```python
from build123d import *

# Parameters (mm, degrees)
ESQUISSE1_R             = 28
BOSS_EXTRU_1_DEPTH      = 7
ESQUISSE2_R             = 3.8
BOSS_EXTRU_2_DEPTH      = 10
ESQUISSE3_R             = 3.05
ENL_V_MAT_EXTRU_1_DEPTH = 18
ESQUISSE4_R             = 2
ESQUISSE5_R             = 5.75
ESQUISSE5_R_2           = 3.8
BOSS_EXTRU_3_DEPTH      = 6
ENL_V_MAT_EXTRU_2_REACH = 30
ESQUISSE6_R             = 1.5


with BuildPart() as part:
    # Esquisse1 → Boss.-Extru.1 (new body)
    with BuildSketch(Plane.XY):
        Circle(ESQUISSE1_R)
    extrude(amount=BOSS_EXTRU_1_DEPTH)

    # Esquisse2 → Boss.-Extru.2 (add)
    with BuildSketch(Plane.XY.offset(7)):
        Circle(ESQUISSE2_R)
    extrude(amount=BOSS_EXTRU_2_DEPTH)

    # Esquisse3 → Enlèv. mat.-Extru.1 (cut, through all)
    with BuildSketch(Plane.XY.offset(17)):
        Circle(ESQUISSE3_R)
    extrude(amount=-ENL_V_MAT_EXTRU_1_DEPTH, mode=Mode.SUBTRACT)

    # Esquisse4 → Enlèvement de matière-Révolution1 (revolve, cut)
    with BuildSketch(Plane(origin=(0, 0, 0), x_dir=(0, 0, -1), z_dir=(1, 0, 0))):
        with Locations((-3.5, 28)):
            Circle(ESQUISSE4_R)
    revolve(axis=Axis((0, 0, 0), (0, 0, 1)), mode=Mode.SUBTRACT)

    # Esquisse5 → Boss.-Extru.3 (add)
    with BuildSketch(Plane.XY.offset(7)):
        Circle(ESQUISSE5_R)
        Circle(ESQUISSE5_R_2, mode=Mode.SUBTRACT)
    extrude(amount=BOSS_EXTRU_3_DEPTH)

    # Esquisse6 → Enlèv. mat.-Extru.2 (cut, up to next)
    with BuildSketch(Plane(origin=(0, 0, 0), x_dir=(1, 0, 0), z_dir=(0, 1, 0)), mode=Mode.PRIVATE) as enl_v_mat_extru_2_sk1:
        with Locations((0, -10)):
            Circle(ESQUISSE6_R)
    enl_v_mat_extru_2_tool1 = extrude(enl_v_mat_extru_2_sk1.sketch, amount=ENL_V_MAT_EXTRU_2_REACH, mode=Mode.PRIVATE) & part.part
    add(enl_v_mat_extru_2_tool1.solids().sort_by_distance((0, 0, 10))[0], mode=Mode.SUBTRACT)


solid = part.part
```
Read the model definition and answer for the solid it produces. Units are mm, in the model's axes. A direction names the side the tool comes from. Give positions to 0.01 mm unless a question says otherwise; leave off trailing zeros. Write each loop counter-clockwise with the first axis right and the second up, starting at its lowest first coordinate (ties: lowest second). Pieces come first, ordered by that corner, then holes. Notation, with made-up numbers: (-36, 8) -> (-28, 8) arc R22 ccw to (-28, 44) -> close; hole circle Ø5 at (84, 13). An arc over 180 degrees is marked (long way). Answer as a JSON object with one key per item and string values.
1) Flat-ended cylindrical pins translate along their axes: pin 1 Ø3.5 at (x, z) = (0, 10) entering from +Y; pin 2 Ø2 at (x, z) = (14.5, 5) entering from +Y; pin 3 Ø10 at (x, y) = (-9, -2) entering from +Z. Find the tip coordinate at first contact, or state that the pin passes through.
Findings below:
{"pin 1": "stops at y = 5.75", "pin 2": "stops at y = 24.46", "pin 3": "stops at z = 13"}
2) For a pull along X with two mould halves and no side action, classify faces 3 (the flat face through (6, 0, 0)), 4 (the cylindrical face through (26.707, 8.41, 0.74)), 5 (the cylindrical face through (1.386, 4.184, 10.575)) as pulls with the +X half, pulls with the -X half, needs draft (parallel to the pull), parting line crosses it, or undercut.
Findings below:
{"face 3": "needs draft", "face 4": "parting line crosses it", "face 5": "undercut"}
3) Straight lines are drawn through the part: probe 1 along Z at (x, y) = (0, 4); probe 2 along Z at (x, y) = (13.5, -9); probe 3 along Y at (x, z) = (0, 6.5). For each, find the intervals that lie inside material, in ascending order. Write a range as from..to.
Findings below:
{"probe 1": "z = 0..8.5, 11.5..13", "probe 2": "z = 0..7", "probe 3": "y = -28..-3.05, 3.05..28"}
4) Section B-B on x = 0 is taken. Write down the section's boundary in (y, z), then the cut area to 3 significant figures.
Findings below:
{"outline": "(-28, 0) -> (-3.05, 0) -> (-3.05, 17) -> (-3.8, 17) -> (-3.8, 13) -> (-5.75, 13) -> (-5.75, 7) -> (-28, 7) -> (-28, 5.5) arc R2 cw to (-28, 1.5) -> close; (3.05, 0) -> (28, 0) -> (28, 1.5) arc R2 cw to (28, 5.5) -> (28, 7) -> (5.75, 7) -> (5.75, 8.5) -> (3.05, 8.5) -> close; (3.05, 11.5) -> (5.75, 11.5) -> (5.75, 13) -> (3.8, 13) -> (3.8, 17) -> (3.05, 17) -> close", "area": "367 mm^2"}
5) A tool of negligible diameter and unlimited length cuts with its end or side. For faces 1 (the flat face through (1, -4, 13)), 2 (the cylindrical face through (25.865, -10.724, 6.24)), from which of +Z, -Z, +X, -X, +Y, -Y can it reach the whole face along a straight path? Write none if from no direction.
Findings below:
{"face 1": "+Z", "face 2": "+Z, -Z"}
6) Section A-A on y = 0 is taken. Write down the section's boundary in (x, z).
Findings below:
{"outline": "(-28, 0) -> (-3.05, 0) -> (-3.05, 17) -> (-3.8, 17) -> (-3.8, 13) -> (-5.75, 13) -> (-5.75, 7) -> (-28, 7) -> (-28, 5.5) arc R2 cw to (-28, 1.5) -> close; (3.05, 0) -> (28, 0) -> (28, 1.5) arc R2 cw to (28, 5.5) -> (28, 7) -> (5.75, 7) -> (5.75, 13) -> (3.8, 13) -> (3.8, 17) -> (3.05, 17) -> close"}
7) Section C-C on z = 7.75 is taken. Write down the section's boundary in (x, y).
Findings below:
{"outline": "circle Ø11.5 at (0, 0); hole circle Ø6.1 at (0, 0)"}
